Verification items for the finished model (mm, model axes). Face numbers are marked on the shaded views. A direction names the side the tool comes from. Round coordinates to 2 decimals unless told otherwise and drop trailing zeros. Write each loop counter-clockwise with the first axis right and the second up, starting at its lowest first coordinate (ties: lowest second). Pieces come first, ordered by that corner, then holes. Notation, with made-up numbers: (85, -4.5) -> (110, -4.5) arc R28 ccw to (110, 24.5) -> close; hole circle Ø11 at (33, 32.5). An arc over 180 degrees is marked (long way). Answer as a JSON object with one key per item and string values. Group by question number.
(1) Set-up check for the marked faces 1 and 2: record each of +Z, -Z, +X, -X, +Y, -Y from which the full face is reachable in a straight line by a thin tool's end or side.
(2) Sectioned sample at C-C on x = -39.5. Record the cut outline in (y, z).
(3) Sectioned sample at B-B on z = -78. Record the cut outline in (x, y), and give its area (3 significant figures).
(4) Sectioned sample at D-D on y = 96. Record the cut outline in (x, z), and give its area (3 significant figures).
(5) Sectioned sample at A-A on y = 37.5. Record the cut outline in (x, z), and give its area (3 significant figures).
(6) Draft check along Z on the marked faces 3, 4 and 5. Enter one of: released by +Z, released by -Z, zero draft, split by the parting line, or undercut.
(7) Scan lines: L1, parallel to X at y = 75.5, z = -52; L2, parallel to Z at x = 243, y = 70; L3, parallel to Y at x = 188.5, z = -75. Record each from-to range of solid material in increasing order. Write a range as from..to.
(8) Gauge pin test, flat ends, axial feed: pin 1 Ø3 at (x, z) = (141.5, -108.5) entering from +Y; pin 2 Ø1.5 at (x, z) = (-198, -107.5) entering from -Y; pin 3 Ø12 at (x, y) = (172, 44) entering from +Z; pin 4 Ø5 at (y, z) = (128.5, -24) entering from -X. Record the tip position at first contact, or that the pin passes through.
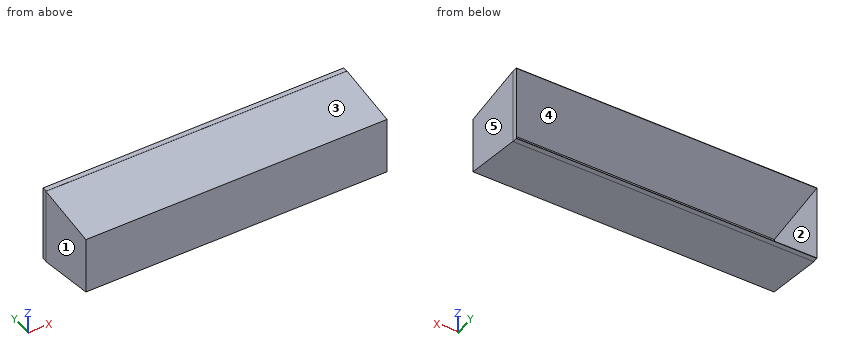
```python
from build123d import *

# Parameters (mm, degrees)
BOSS_EXTRUDE1_DEPTH = 300
SKETCH2_W           = 616.91666666
SKETCH2_H           = 169.999999994
BOSS_EXTRUDE2_DEPTH = 5
CUT_EXTRUDE1_START  = -300
CUT_EXTRUDE1_DEPTH  = 299
SKETCH4_W           = 616.91666666
SKETCH4_H           = 10
CUT_EXTRUDE2_DEPTH  = 9
SKETCH5_W           = 616.91666666
SKETCH5_H           = 10
CUT_EXTRUDE3_DEPTH  = 9
SKETCH6_W           = 151.999999994
SKETCH6_H           = 10
CUT_EXTRUDE4_DEPTH  = 9
SKETCH7_W           = 151.999999994
SKETCH7_H           = 10
CUT_EXTRUDE5_DEPTH  = 9


with BuildPart() as part:
    # Sketch1 → Boss-Extrude1 (new, symmetric)
    with BuildSketch(Plane(origin=(0, 0, 0), x_dir=(0, 0, -1), z_dir=(1, 0, 0))):
        Polygon((0, 0), (113, 0), (133.041666667, 130), (-20.041666667, 130), align=None)
    extrude(amount=BOSS_EXTRUDE1_DEPTH, both=True)

    # Sketch2 → Boss-Extrude2 (add, symmetric)
    with BuildSketch(Plane(origin=(0, 130, 0), x_dir=(1, 0, 0), z_dir=(0, 1, 0))):
        with Locations((0, 56.5)):
            Rectangle(SKETCH2_W, SKETCH2_H)
    extrude(amount=BOSS_EXTRUDE2_DEPTH, both=True)

    # Sketch3 → Cut-Extrude1 (cut, symmetric)
    with BuildSketch(Plane.ZY.offset(300).offset(CUT_EXTRUDE1_START)):
        Polygon((-131.788872207, 135), (18.788872207, 135), (-1.71529446, 2), (-111.28470554, 2), align=None)
    extrude(amount=CUT_EXTRUDE1_DEPTH, both=True, mode=Mode.SUBTRACT)

    # Sketch4 → Cut-Extrude2 (cut)
    with BuildSketch(Plane(origin=(0, 0, -141.499999997), x_dir=(-1, 0, 0), z_dir=(0, 0, -1))):
        with Locations((0, 130)):
            Rectangle(SKETCH4_W, SKETCH4_H)
    extrude(amount=-CUT_EXTRUDE2_DEPTH, mode=Mode.SUBTRACT)

    # Sketch5 → Cut-Extrude3 (cut)
    with BuildSketch(Plane.XY.offset(28.499999997)):
        with Locations((0, 130)):
            Rectangle(SKETCH5_W, SKETCH5_H)
    extrude(amount=-CUT_EXTRUDE3_DEPTH, mode=Mode.SUBTRACT)

    # Sketch6 → Cut-Extrude4 (cut)
    with BuildSketch(Plane.ZY.offset(308.45833333)):
        with Locations((-56.5, 130)):
            Rectangle(SKETCH6_W, SKETCH6_H)
    extrude(amount=-CUT_EXTRUDE4_DEPTH, mode=Mode.SUBTRACT)

    # Sketch7 → Cut-Extrude5 (cut)
    with BuildSketch(Plane(origin=(308.45833333, 0, 0), x_dir=(0, 0, -1), z_dir=(1, 0, 0))):
        with Locations((56.5, 130)):
            Rectangle(SKETCH7_W, SKETCH7_H)
    extrude(amount=-CUT_EXTRUDE5_DEPTH, mode=Mode.SUBTRACT)


solid = part.part
```
Computed values:
{
 "1": {"face 1": "+Z, -Z, -X, +Y, -Y", "face 2": "+Y"},
 "2": {"outline": "(0, -113) -> (125, -132.27) -> (125, -132.5) -> (135, -132.5) -> (135, -131.79) -> (2, -111.28) -> (2, -1.72) -> (135, 18.79) -> (135, 19.5) -> (125, 19.5) -> (125, 19.27) -> (0, 0) -> close"},
 "3": {"outline": "(-300, 0) -> (300, 0) -> (300, 125) -> (299.46, 125) -> (299.46, 135) -> (299, 135) -> (299, 2) -> (-299, 2) -> (-299, 135) -> (-299.46, 135) -> (-299.46, 125) -> (-300, 125) -> close", "area": "1,460 mm2"},
 "4": {"outline": "(-300, -127.8) -> (300, -127.8) -> (300, 14.8) -> (-300, 14.8) -> close; hole (-299, -125.78) -> (299, -125.78) -> (299, 12.78) -> (-299, 12.78) -> close", "area": "2,710 mm2"},
 "5": {"outline": "(-300, -118.78) -> (300, -118.78) -> (300, 5.78) -> (-300, 5.78) -> close; hole (-299, -116.76) -> (299, -116.76) -> (299, 3.76) -> (-299, 3.76) -> close", "area": "2,670 mm2"},
 "6": {"face 3": "released by +Z", "face 4": "undercut", "face 5": "zero draft"},
 "7": {"L1": "-300..-299, 299..300", "L2": "-123.79..-121.77, 8.77..10.79", "L3": "0..2"},
 "8": {"pin 1": "y = 2", "pin 2": "y = 0", "pin 3": "z = 7.71", "pin 4": "x = -299.46"}
}
